For this review, take the finished solid that the model builds, in its own axes (mm). Face numbers are marked on the shaded views. A direction names the side the tool comes from. Coordinates: 2 decimals unless noted, no trailing zeros. Write each loop counter-clockwise with the first axis right and the second up, starting at its lowest first coordinate (ties: lowest second). Pieces come first, ordered by that corner, then holes. Notation, with made-up numbers: (-1.75, 10) -> (56.25, 10) arc R24 ccw to (56.25, 22) -> close; hole circle Ø10 at (88.5, -29). An arc over 180 degrees is marked (long way). Put each result on its own line as item: value. Start each with the question number.
Item 1: To check wall thickness, follow L1, parallel to Y at x = 0, z = 3.95; L2, parallel to Y at x = -4, z = 1.55; L3, parallel to Y at x = 1, z = 1.75. State the ranges of each line that lie inside material, in increasing order.
Item 2: Insertion check: P1, Ø1, axis at x = -3.5, z = 3.5, coming from the -Y side; P2, Ø2.5, axis at x = -9.5, z = 2.5, coming from the -Y side; P3, Ø1.5, axis at y = -3, z = 2, coming from the -X side; P4, Ø4, axis at x = 0, y = 0, coming from the +Z side. Each pin has a flat end and moves straight along its axis. Give the tip position at first contact, or say it passes through.
Item 3: Consider section D-D on x = -7. Give the boundary of the cut face in (y, z), and give its area (3 significant figures).
Item 4: For the marked faces 1 and 2, list the 3-axis set-ups (+Z, -Z, +X, -X, +Y, -Y) from which the entire face can be reached by the end or side of a thin tool; tool diameter is ignored.
Item 5: Consider section A-A on z = 2.95. Give the boundary of the cut face in (x, y), and give its area (3 significant figures).
Item 6: Consider section B-B on y = 0. Give the boundary of the cut face in (x, z), and give its area (3 significant figures).
Autodesk Inventor part; units mm, degrees
sketch "Sketch1" plane through (0, 0, 0) normal (0, 0, 1) x (1, 0, 0)
  line L0 (-5.7775, 0) -> (5.7775, 0) construction
  line L1 (4.5, 7.5) -> (-12.5, 7.5)
  line L2 (-12.5, 7.5) -> (4.5, 7.5)
  line L3 (4.5, 7.5) -> (7.5, 4.5)
  line L4 (4.5, 7.5) -> (7.5, 4.5)
  line L5 (7.5, 4.5) -> (7.5, -12.5)
  line L6 (7.5, 4.5) -> (7.5, -12.5)
  line L7 (2.5, -12.5) -> (7.5, -12.5)
  line L8 (7.5, -12.5) -> (2.5, -12.5)
  line L9 (-7.5, -7.5) -> (2.5, -7.5)
  line L10 (2.5, -12.5) -> (2.5, -7.5)
  line L11 (2.5, -7.5) -> (-7.5, -7.5)
  line L12 (-7.5, 2.5) -> (-7.5, -7.5)
  line L13 (-7.5, -7.5) -> (-7.5, 2.5)
  line L14 (-7.5, 2.5) -> (-12.5, 2.5)
  line L15 (-7.5, 2.5) -> (-12.5, 2.5)
  line L16 (-12.5, 2.5) -> (-12.5, 7.5)
extrude "Extrusion1" add sketch "Sketch1" along normal blind 5
sketch "Sketch2" plane through (0, 0, 5) normal (0, 0, 1) x (1, 0, 0)
  circle A0 centre (0, 0) radius 2.25
  dimension "d2" = 4.5
extrude "Extrusion2" cut sketch "Sketch2" against normal blind 5
properties part number "bevestiging deksel zonder moer" material "S235"
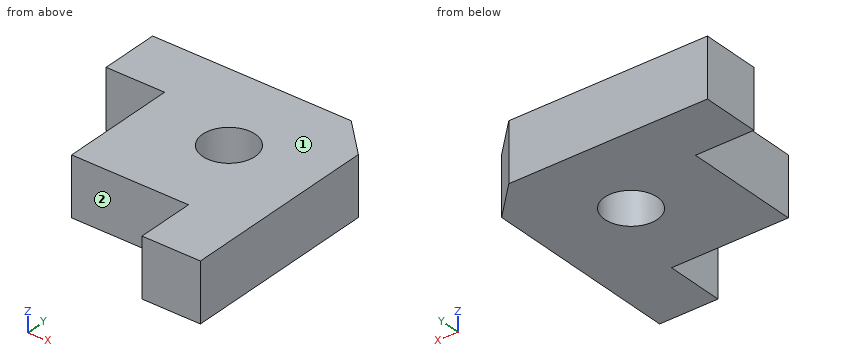
Return value:
1. L1: -7.5 to -2.25, 2.25 to 7.5
1. L2: -7.5 to 7.5
1. L3: -7.5 to -2.02, 2.02 to 7.5
2. P1: y = -7.5
2. P2: y = 2.5
2. P3: x = -7.5
2. P4: through
3. outline: (-7.5, 0) -> (7.5, 0) -> (7.5, 5) -> (-7.5, 5) -> close
3. area: 75.0 mm^2
4. face 1: +Z, +X, -X, +Y, -Y
4. face 2: +Z, -Z, -X, -Y
5. outline: (-12.5, 2.5) -> (-7.5, 2.5) -> (-7.5, -7.5) -> (2.5, -7.5) -> (2.5, -12.5) -> (7.5, -12.5) -> (7.5, 4.5) -> (4.5, 7.5) -> (-12.5, 7.5) -> close; hole circle Ø4.5 at (0, 0)
5. area: 255 mm^2
6. outline: (-7.5, 0) -> (-2.25, 0) -> (-2.25, 5) -> (-7.5, 5) -> close; (2.25, 0) -> (7.5, 0) -> (7.5, 5) -> (2.25, 5) -> close
6. area: 52.5 mm^2
